```python
from build123d import *

# Parameters (mm, degrees)
SKETCH5_W                                      = 60
SKETCH5_H                                      = 30
BOSS_EXTRUDE3_DEPTH                            = 40
SKETCH7_W                                      = 40
SKETCH7_H                                      = 20
CUT_EXTRUDE1_DEPTH                             = 15
FILLET1_R                                      = 3
FILLET2_R                                      = 3
FILLET3_R                                      = 3
FILLET4_R                                      = 3
SKETCH9_W                                      = 30
SKETCH9_H                                      = 5
BOSS_EXTRUDE4_DEPTH                            = 7
SKETCH10_W                                     = 30
SKETCH10_H                                     = 5
BOSS_EXTRUDE5_DEPTH                            = 7
SKETCH12_R                                     = 2
CUT_EXTRUDE2_DEPTH                             = 10
SKETCH13_W                                     = 64
SKETCH13_H                                     = 20
CUT_EXTRUDE3_DEPTH                             = 1.5
F_2_56_TAPPED_HOLE2_D                          = 1.778
F_2_56_TAPPED_HOLE2_DEPTH                      = 15
F_2_56_TAPPED_HOLE2_TIP                        = 0.53416509
F_2_56_TAPPED_HOLE3_D                          = 1.778
F_2_56_TAPPED_HOLE3_DEPTH                      = 15
F_2_56_TAPPED_HOLE3_TIP                        = 0.53416509
CBORE_FOR_2_SOCKET_HEAD_CAP_SCREW3_D           = 2.4384
CBORE_FOR_2_SOCKET_HEAD_CAP_SCREW3_DEPTH       = 15
CBORE_FOR_2_SOCKET_HEAD_CAP_SCREW3_CBORE_D     = 4.7625
CBORE_FOR_2_SOCKET_HEAD_CAP_SCREW3_CBORE_DEPTH = 2.1844
CBORE_FOR_2_SOCKET_HEAD_CAP_SCREW3_TIP         = 0.732569267
F_8_32_TAPPED_HOLE1_D                          = 3.4544
F_8_32_TAPPED_HOLE1_DEPTH                      = 11
F_8_32_TAPPED_HOLE1_TIP                        = 1.037806461
F_0_535_40_TAPPED_HOLE1_D                      = 13.2842
SKETCH30_R                                     = 1.5
SKETCH30_R_2                                   = 3
CUT_EXTRUDE5_DEPTH                             = 10
CBORE_FOR_2_SOCKET_HEAD_CAP_SCREW4_D           = 2.4384
CBORE_FOR_2_SOCKET_HEAD_CAP_SCREW4_CBORE_D     = 4.7625
CBORE_FOR_2_SOCKET_HEAD_CAP_SCREW4_CBORE_DEPTH = 2.1844


with BuildPart() as part:
    # Sketch5 → Boss-Extrude3 (new body)
    with BuildSketch(Plane(origin=(0, 0, 0), x_dir=(1, 0, 0), z_dir=(0, 1, 0))):
        Rectangle(SKETCH5_W, SKETCH5_H)
    extrude(amount=BOSS_EXTRUDE3_DEPTH)

    # Sketch7 → Cut-Extrude1 (cut)
    with BuildSketch(Plane(origin=(0, 0, -15), x_dir=(-1, 0, 0), z_dir=(0, 0, -1))):
        with Locations((0, 20)):
            Rectangle(SKETCH7_W, SKETCH7_H)
    extrude(amount=-CUT_EXTRUDE1_DEPTH, mode=Mode.SUBTRACT)

    # Fillet1
    fillet1_edges = [part.edges().sort_by_distance(p)[0] for p in [
        (20, 10, -7.5),
    ]]
    fillet(fillet1_edges, radius=FILLET1_R)

    # Fillet2
    fillet2_edges = [part.edges().sort_by_distance(p)[0] for p in [
        (-20, 10, -7.5),
    ]]
    fillet(fillet2_edges, radius=FILLET2_R)

    # Fillet3
    fillet3_edges = [part.edges().sort_by_distance(p)[0] for p in [
        (-20, 30, -7.5),
    ]]
    fillet(fillet3_edges, radius=FILLET3_R)

    # Fillet4
    fillet4_edges = [part.edges().sort_by_distance(p)[0] for p in [
        (20, 30, -7.5),
    ]]
    fillet(fillet4_edges, radius=FILLET4_R)

    # Sketch9 → Boss-Extrude4 (add)
    with BuildSketch(Plane.ZY.offset(30)):
        with Locations((0, 2.5)):
            Rectangle(SKETCH9_W, SKETCH9_H)
    extrude(amount=BOSS_EXTRUDE4_DEPTH)

    # Sketch10 → Boss-Extrude5 (add)
    with BuildSketch(Plane(origin=(30, 0, 0), x_dir=(0, 0, -1), z_dir=(1, 0, 0))):
        with Locations((0, 2.5)):
            Rectangle(SKETCH10_W, SKETCH10_H)
    extrude(amount=BOSS_EXTRUDE5_DEPTH)

    # Sketch12 → Cut-Extrude2 (cut)
    with BuildSketch(Plane.ZY.offset(30)):
        with Locations((-7.531524718, 22.710545663)):
            Circle(SKETCH12_R)
    extrude(amount=-CUT_EXTRUDE2_DEPTH, mode=Mode.SUBTRACT)

    # Sketch13 → Cut-Extrude3 (cut)
    with BuildSketch(Plane(origin=(0, 0, 0), x_dir=(-1, 0, 0), z_dir=(0, -1, 0))):
        Rectangle(SKETCH13_W, SKETCH13_H)
    extrude(amount=-CUT_EXTRUDE3_DEPTH, mode=Mode.SUBTRACT)

    # #2-56 Tapped Hole2
    with Locations(Plane(origin=(25, 36, -15), x_dir=(-1, 0, 0), z_dir=(0, 0, -1))):
        with Locations((0, 0), (0, -32), (50, -32)):
            Hole(F_2_56_TAPPED_HOLE2_D / 2, depth=F_2_56_TAPPED_HOLE2_DEPTH)
            with Locations((0, 0, -(F_2_56_TAPPED_HOLE2_DEPTH + F_2_56_TAPPED_HOLE2_TIP / 2))):  # 118° drill point
                Cone(0, F_2_56_TAPPED_HOLE2_D / 2, F_2_56_TAPPED_HOLE2_TIP, mode=Mode.SUBTRACT)

    # #2-56 Tapped Hole3
    with Locations(Plane(origin=(-25, 36, -15), x_dir=(-1, 0, 0), z_dir=(0, 0, -1))):
        with Locations((0, 0)):
            Hole(F_2_56_TAPPED_HOLE3_D / 2, depth=F_2_56_TAPPED_HOLE3_DEPTH)
            with Locations((0, 0, -(F_2_56_TAPPED_HOLE3_DEPTH + F_2_56_TAPPED_HOLE3_TIP / 2))):  # 118° drill point
                Cone(0, F_2_56_TAPPED_HOLE3_D / 2, F_2_56_TAPPED_HOLE3_TIP, mode=Mode.SUBTRACT)

    # CBORE for #2 Socket Head Cap Screw3
    with Locations(Plane(origin=(0, 5, 0), x_dir=(1, 0, 0), z_dir=(0, 1, 0))):
        with Locations((-33.5, 8), (-33.5, -8)):
            CounterBoreHole(CBORE_FOR_2_SOCKET_HEAD_CAP_SCREW3_D / 2, CBORE_FOR_2_SOCKET_HEAD_CAP_SCREW3_CBORE_D / 2, CBORE_FOR_2_SOCKET_HEAD_CAP_SCREW3_CBORE_DEPTH, depth=CBORE_FOR_2_SOCKET_HEAD_CAP_SCREW3_DEPTH)
            with Locations((0, 0, -(CBORE_FOR_2_SOCKET_HEAD_CAP_SCREW3_DEPTH + CBORE_FOR_2_SOCKET_HEAD_CAP_SCREW3_TIP / 2))):  # 118° drill point
                Cone(0, CBORE_FOR_2_SOCKET_HEAD_CAP_SCREW3_D / 2, CBORE_FOR_2_SOCKET_HEAD_CAP_SCREW3_TIP, mode=Mode.SUBTRACT)

    # #8-32 Tapped Hole1
    with Locations(Plane.XY.offset(15)):
        with Locations((-20, 30), (-20, 10), (20, 10), (20, 30)):
            Hole(F_8_32_TAPPED_HOLE1_D / 2, depth=F_8_32_TAPPED_HOLE1_DEPTH)
            with Locations((0, 0, -(F_8_32_TAPPED_HOLE1_DEPTH + F_8_32_TAPPED_HOLE1_TIP / 2))):  # 118° drill point
                Cone(0, F_8_32_TAPPED_HOLE1_D / 2, F_8_32_TAPPED_HOLE1_TIP, mode=Mode.SUBTRACT)

    # 0.535-40 Tapped Hole1 (through all)
    with Locations(Plane(origin=(0, 20, 0), x_dir=(-1, 0, 0), z_dir=(0, 0, -1))):
        with Locations((0, 0)):
            Hole(F_0_535_40_TAPPED_HOLE1_D / 2)

    # Sketch30 → Cut-Extrude5 (cut)
    with BuildSketch(Plane(origin=(0, 0, 0), x_dir=(-1, 0, 0), z_dir=(0, 0, -1))):
        with Locations((-12.5, 20)):
            Circle(SKETCH30_R)
        with Locations((12.5, 20)):
            Circle(SKETCH30_R_2)
    extrude(amount=-CUT_EXTRUDE5_DEPTH, mode=Mode.SUBTRACT)

    # CBORE for #2 Socket Head Cap Screw4 (through all)
    with Locations(Plane(origin=(33.5, 5, 8), x_dir=(0, 0, 1), z_dir=(0, 1, 0))):
        with Locations((0, 0), (-16, 0)):
            CounterBoreHole(CBORE_FOR_2_SOCKET_HEAD_CAP_SCREW4_D / 2, CBORE_FOR_2_SOCKET_HEAD_CAP_SCREW4_CBORE_D / 2, CBORE_FOR_2_SOCKET_HEAD_CAP_SCREW4_CBORE_DEPTH)


solid = part.part
```
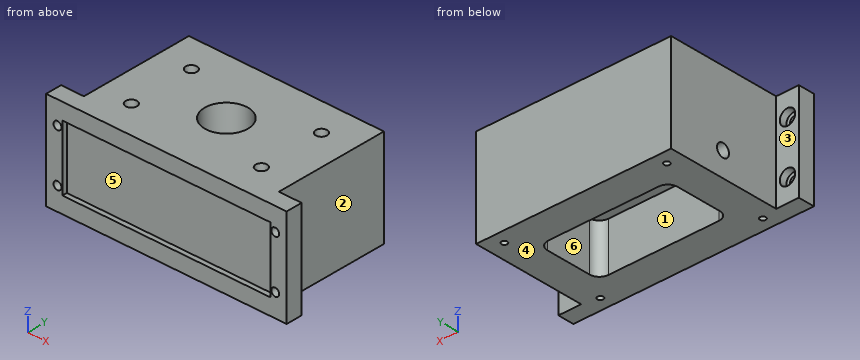
Verification items for the finished model (mm, model axes). Face numbers are marked on the shaded views. A direction names the side the tool comes from. Coordinates: 2 decimals unless noted, no trailing zeros. Write each loop counter-clockwise with the first axis right and the second up, starting at its lowest first coordinate (ties: lowest second). Pieces come first, ordered by that corner, then holes. Notation, with made-up numbers: M 38.25,-36.75 L 80.25,-36.75 A14 ccw 80.25,-15.75 Z; hole C -29,11.25 d11. An arc over 180 degrees is marked long. Answer as a JSON object with one key per item and string values. Group by question number.
(1) Cross-section at D-D, the plane y = 25.5. Record the cut outline in (x, z), and give its area (3 significant figures).
(2) Cross-section at A-A, the plane x = 0. Record the cut outline in (y, z).
(3) Cross-section at B-B, the plane z = -11.25. Record the cut outline in (x, y), and give its area (3 significant figures).
(4) Tool access check on the marked faces 1, 2 and 3. Record the directions out of +Z, -Z, +X, -X, +Y, -Y that give a thin tool (end or side, any length) a straight path to the whole face; none if there is none.
(5) Gauge pin test, flat ends, axial feed: pin 1 (5.5 mm diameter, centred on x = -33.5, z = -0.5, fed in from +Y); pin 2 (8 mm diameter, centred on x = 17.5, z = -3, fed in from -Y); pin 3 (15 mm diameter, centred on y = 17.5, z = 6, fed in from +X); pin 4 (4.5 mm diameter, centred on x = 20, y = 30, fed in from +Z). Record the tip position at first contact, or that the pin passes through.
(6) Material ranges on line 1 (X direction, y = 30, z = 7); line 2 (X direction, y = 22, z = 5.5); line 3 (X direction, y = 4, z = -8.5), recorded low to high.
(7) Release check for a two-part mould opening along Z. For the marked faces 4, 5 and 6 record: +Z half, -Z half, draft (parallel to the pull), parting line (faces both ways), or undercut.
(8) Cross-section at C-C, the plane x = -12.5. Record the cut outline in (y, z), and give its area (3 significant figures).
Reply:
{
 "1": {"outline": "M -30,-15 L -20,-15 L -20,0 L -3.72,0 L -3.72,15 L -30,15 Z; M 3.72,0 L 20,0 L 20,-15 L 30,-15 L 30,15 L 3.72,15 Z", "area": "1,090 mm²"},
 "2": {"outline": "M 0,-15 L 10,-15 L 10,0 L 13.36,0 L 13.36,15 L 0,15 L 0,10 L 1.5,10 L 1.5,-10 L 0,-10 Z; M 26.64,0 L 30,0 L 30,-15 L 40,-15 L 40,15 L 26.64,15 Z"},
 "3": {"outline": "M -37,0 L 37,0 L 37,5 L 30,5 L 30,40 L -30,40 L -30,5 L -37,5 Z; hole C -25,4 d1.78; hole C -25,36 d1.78; hole M -20,13 A3 ccw -17,10 L 17,10 A3 ccw 20,13 L 20,27 A3 ccw 17,30 L -17,30 A3 ccw -20,27 Z; hole C 25,4 d1.78; hole C 25,36 d1.78", "area": "1,670 mm²"},
 "4": {"face 1": "-Z", "face 2": "+Z, -Z, +X, +Y", "face 3": "+Z, -Z, -X, +Y"},
 "5": {"pin 1": "y = 5", "pin 2": "y = 1.5", "pin 3": "x = 30", "pin 4": "z = 15"},
 "6": {"line 1": "-30 to -21.73, -18.27 to 18.27, 21.73 to 30", "line 2": "-30 to -14.74, -10.26 to -6.33, 6.33 to 30", "line 3": "-37 to -35.83, -31.17 to -25.89, -24.11 to 24.11, 25.89 to 31.17, 35.83 to 37"},
 "7": {"face 4": "-Z half", "face 5": "undercut", "face 6": "draft"},
 "8": {"outline": "M 0,-15 L 10,-15 L 10,0 L 17,0 L 17,10 L 23,10 L 23,0 L 30,0 L 30,-15 L 40,-15 L 40,15 L 0,15 L 0,10 L 1.5,10 L 1.5,-10 L 0,-10 Z", "area": "810 mm²"}
}
